from build123d import *

# Parameters (mm, degrees)
F0_R          = 138.6669495236
F1_DEPTH      = 25.4
F2_W          = 85.052728653
F2_H          = 27.0034535788
F3_DEPTH      = 508
F3_DEPTH_BACK = 25.4
F4_DEPTH      = 508


with BuildPart() as f1:
    # F0 (on Top) → F1 (new body)
    with BuildSketch(Plane.XY):
        Circle(F0_R)
    extrude(amount=F1_DEPTH)

    # F2 (on Front) → F3 (join, two sides)
    with BuildSketch(Plane.XZ) as f3_sk:
        with Locations((-5.2903704345, 6.888640346)):
            Rectangle(F2_W, F2_H)
    extrude(amount=-F3_DEPTH)
    extrude(f3_sk.sketch, amount=F3_DEPTH_BACK)

    # F4 (add): a face of the model
    f4_faces = [f1.faces().sort_by_distance(p)[0] for p in [
        (-5.2903704345, -25.4, -3.3065432217),
    ]]
    extrude(f4_faces, amount=F4_DEPTH)


solid = f1.part
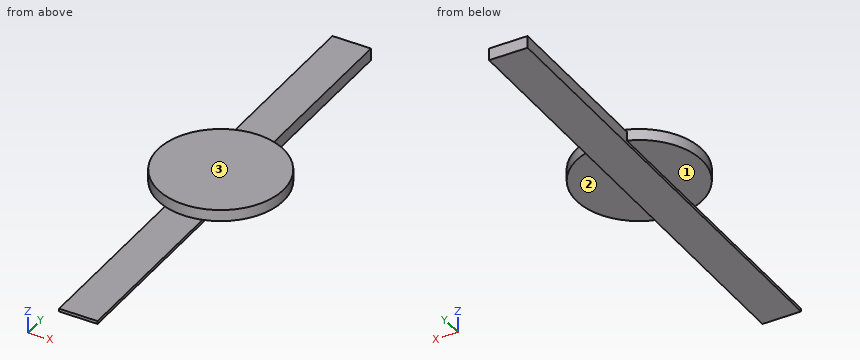
The listing builds one solid part. Answer for the finished solid, in the listing's coordinates (mm). Face numbers are marked on the shaded views. A direction names the side the tool comes from. Round coordinates to 2 decimals unless told otherwise and drop trailing zeros. Write each loop counter-clockwise with the first axis right and the second up, starting at its lowest first coordinate (ties: lowest second). Pieces come first, ordered by that corner, then holes. Notation, with made-up numbers: M 44.25,61 L 48.25,61 A34 cw 48.25,95 Z; hole C 21.5,-2 d4. An arc over 180 degrees is marked long. Write each question's results on one line, items separated by ' | '. Start each with the question number.
(1) Find the intervals of material crossed by line 1 (Z direction, x = 23, y = -177); line 2 (Z direction, x = -57.5, y = 71); line 3 (Y direction, x = -3, z = 22), in increasing order.
(2) For the marked faces 1, 2 and 3, determine the directions among +Z, -Z, +X, -X, +Y, -Y from which every point of the face is accessible in a straight line to the end or side of a thin tool.
(3) The part is cut by section D-D, the plane y = -269. Write down the section's boundary in (x, z), and give its area (3 significant figures).
(4) The part is cut by section A-A, the plane y = 0. Write down the section's boundary in (x, z).
(5) The part is cut by section B-B, the plane x = 0. Write down the section's boundary in (y, z).
(6) The part is cut by section C-C, the plane z = 7.5. Write down the section's boundary in (x, y).
(7) Each of these flat-tipped pins is pushed along its axis until it touches: P1, Ø3, axis at x = 40, y = -116.5, coming from the -Z side; P2, Ø8, axis at y = 155, z = 3, coming from the -X side; P3, Ø5, axis at y = 371.5, z = 16.5, coming from the +X side. Where does it stop, or does it pass through?
Worked answers:
1) line 1: z = -6.61 to 0 | line 2: z = 0 to 25.4 | line 3: y = -138.63 to 138.63
2) face 1: -Z, -X, +Y, -Y | face 2: -Z, +X, +Y, -Y | face 3: +Z, +X, -X, +Y, -Y
3) outline: M -47.82,-6.61 L 37.24,-6.61 L 37.24,0 L -47.82,0 Z | area: 562 mm²
4) outline: M -138.67,0 L -47.82,0 L -47.82,-6.61 L 37.24,-6.61 L 37.24,0 L 138.67,0 L 138.67,25.4 L -138.67,25.4 Z
5) outline: M -533.4,-6.61 L 508,-6.61 L 508,20.39 L 138.67,20.39 L 138.67,25.4 L -138.67,25.4 L -138.67,0 L -533.4,0 Z
6) outline: M -47.82,130.16 A138.67 ccw long 37.24,133.57 L 37.24,508 L -47.82,508 Z
7) P1: stops at z = 0 | P2: stops at x = -47.82 | P3: stops at x = 37.24
